from build123d import *

# Parameters (mm, degrees)
SKETCH_1_W               = 12
SKETCH_1_H               = 12
EXTRUDE_1_DEPTH          = 12
SKETCH_2_R               = 2
CUT_EXTRUDE_1_DEPTH      = 2
PATTERN_CIRCULAR_1_COUNT = 4


with BuildPart() as part:
    # Sketch 1 → Extrude 1 (new body)
    with BuildSketch(Plane(origin=(0, 0, 0), x_dir=(1, 0, 0), z_dir=(0, 1, 0))):
        Rectangle(SKETCH_1_W, SKETCH_1_H)
    extrude(amount=EXTRUDE_1_DEPTH)

    # Sketch 2 → Cut-Extrude 1 (cut)
    with BuildSketch(Plane.XY.offset(6)):
        with Locations((0, 6)):
            Circle(SKETCH_2_R)
    cut_extrude_1 = extrude(amount=-CUT_EXTRUDE_1_DEPTH, mode=Mode.SUBTRACT)

    # Pattern Circular 1: Cut-Extrude 1 ×4 about axis
    pattern_circular_1_axis = Axis((0, 0, 0), (0, 1, 0))
    for i in range(1, PATTERN_CIRCULAR_1_COUNT):
        add(cut_extrude_1.rotate(pattern_circular_1_axis, i * 360 / PATTERN_CIRCULAR_1_COUNT), mode=Mode.SUBTRACT)


solid = part.part
Can you work these out from the model? Positions are in its coordinate system, mm. A direction names the side the tool comes from. Round coordinates to 2 decimals unless told otherwise and drop trailing zeros. Write each loop counter-clockwise with the first axis right and the second up, starting at its lowest first coordinate (ties: lowest second). Pieces come first, ordered by that corner, then holes. Notation, with made-up numbers: M 56,8.25 L 65,8.25 A16 ccw 65,15.25 Z; hole C 50.25,56.5 d5. An arc over 180 degrees is marked long. Use CSV: the item, a comma, the result in double quotes.
(1) Imagine slicing it at D-D (z = 0). Write out the boundary of the cut face in (x, y).
Check values:
outline,"M -6,0 L 6,0 L 6,4 L 4,4 L 4,8 L 6,8 L 6,12 L -6,12 L -6,8 L -4,8 L -4,4 L -6,4 Z"
(2) We'd pull the mould along X, two halves only. Please class faces 1 (the flat face through (0, 3, 6)), 2 (the flat face through (4, 6, 0)), 3 (the flat face through (-4, 6, 0)), 4 (the cylindrical face through (0, 8, -5)): +X half, -X half, draft (parallel to the pull), parting line (faces both ways), or undercut.
Check values:
face 1,"draft"
face 2,"+X half"
face 3,"-X half"
face 4,"undercut"
(3) Imagine slicing it at C-C (y = 6). Write out the boundary of the cut face in (x, z), plus the area to 3 significant figures.
Check values:
outline,"M -6,-6 L -2,-6 L -2,-4 L 2,-4 L 2,-6 L 6,-6 L 6,-2 L 4,-2 L 4,2 L 6,2 L 6,6 L 2,6 L 2,4 L -2,4 L -2,6 L -6,6 L -6,2 L -4,2 L -4,-2 L -6,-2 Z"
area,"112 mm^2"
(4) Imagine slicing it at A-A (z = 4.5). Write out the boundary of the cut face in (x, y).
Check values:
outline,"M -6,0 L 6,0 L 6,12 L -6,12 Z; hole C 0,6 d4"
(5) Imagine slicing it at B-B (x = 0). Write out the boundary of the cut face in (y, z).
Check values:
outline,"M 0,-6 L 4,-6 L 4,-4 L 8,-4 L 8,-6 L 12,-6 L 12,6 L 8,6 L 8,4 L 4,4 L 4,6 L 0,6 Z"
(6) On a 3-axis mill with a long thin cutter (end or side, diameter ignored), from which of +Z, -Z, +X, -X, +Y, -Y can I reach the whole of each face in a straight line? I mean faces 5 (the cylindrical face through (-5, 8, 0)), 6 (the flat face through (0, 6, 4)), 7 (the flat face through (0, 6, -4)), 8 (the cylindrical face through (5, 8, 0)). Say none if no direction works.
Check values:
face 5,"-X"
face 6,"+Z"
face 7,"-Z"
face 8,"+X"
(7) I need wall thicknesses on line 1 along Y through (x, z) = (0, 5.55); line 2 along X through (y, z) = (4.75, 4.5); line 3 along Z through (x, y) = (0.75, 5). Which ranges of each line are inside material? Lowest first, please.
Check values:
line 1,"0 to 4, 8 to 12"
line 2,"-6 to -1.56, 1.56 to 6"
line 3,"-4 to 4"
(8) I'm going to push flat-ended pins straight in: pin 1 (3 mm diameter, centred on y = 6, z = 0, fed in from -X); pin 2 (3 mm diameter, centred on x = 0, y = 6, fed in from +Z); pin 3 (2 mm diameter, centred on y = 6, z = 0, fed in from +X). Where does each tip first touch, or does it pass through?
Check values:
pin 1,"x = -4"
pin 2,"z = 4"
pin 3,"x = 4"
